Model file for the job. Use its own axes, mm. Face numbers are marked on the shaded views. A direction names the side the tool comes from. Give positions to 0.01 mm unless a question says otherwise; leave off trailing zeros. Order: outer loops, then holes, each group sorted by start corner. A loop starts at its lowest first (then second) coordinate and runs counter-clockwise, first axis right, second up. Notation, with made-up numbers: (87.25, -15.75) - (112.25, -15.75) arc R29 ccw to (112.25, 21.25) - close; hole circle Ø5 at (42, 80.25). An arc over 180 degrees is marked (long way). Return JSON: item names as keys, results as strings. Group by question number.
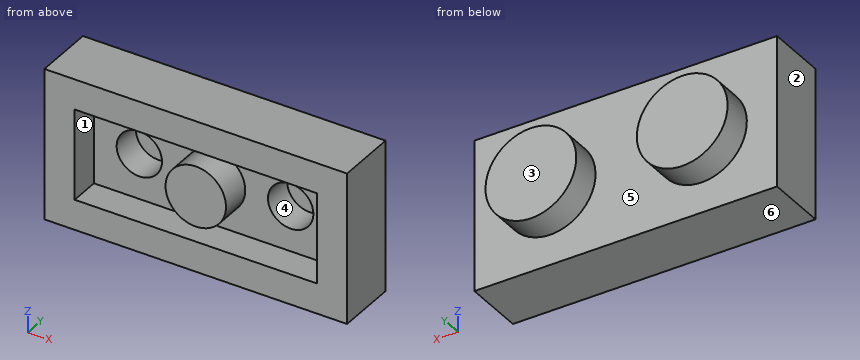
from build123d import *

# Parameters (mm, degrees)
SKETCH1_R           = 1.5
SKETCH1_R_2         = 0.75
BOSS_EXTRUDE1_DEPTH = 2
SKETCH1_3_W         = 10
SKETCH1_3_H         = 5
BOSS_EXTRUDE2_DEPTH = 1
SKETCH1_4_R         = 0.75
CUT_EXTRUDE1_DEPTH  = 1
SKETCH1_5_W         = 10
SKETCH1_5_H         = 5
SKETCH1_5_W_2       = 8
SKETCH1_5_H_2       = 3
SKETCH1_5_R         = 1
BOSS_EXTRUDE3_DEPTH = 1


with BuildPart() as part:
    # Sketch1 → Boss-Extrude1 (new body)
    with BuildSketch(Plane(origin=(0, 0, 0), x_dir=(1, 0, 0), z_dir=(0, 1, 0))):
        with Locations(Location((-2.5, 0, 0), (0, 0, 270))):
            Circle(SKETCH1_R)
        with Locations((-2.5, 0)):
            Circle(SKETCH1_R_2, mode=Mode.SUBTRACT)
        with Locations((-2.5, 0)):
            Circle(SKETCH1_R_2)
        with Locations(Location((2.5, 0, 0), (0, 0, 270))):
            Circle(SKETCH1_R)
        with Locations((2.5, 0)):
            Circle(SKETCH1_R_2, mode=Mode.SUBTRACT)
        with Locations((2.5, 0)):
            Circle(SKETCH1_R_2)
    extrude(amount=BOSS_EXTRUDE1_DEPTH)

    # Sketch1_3 → Boss-Extrude2 (add)
    with BuildSketch(Plane(origin=(0, 0, 0), x_dir=(1, 0, 0), z_dir=(0, 1, 0))):
        Rectangle(SKETCH1_3_W, SKETCH1_3_H)
    extrude(amount=BOSS_EXTRUDE2_DEPTH)

    # Sketch1_4 → Cut-Extrude1 (cut)
    with BuildSketch(Plane(origin=(0, 0, 0), x_dir=(1, 0, 0), z_dir=(0, 1, 0))):
        with Locations(Location((-2.5, 0, 0), (0, 0, 270))):
            Circle(SKETCH1_4_R)
        with Locations(Location((2.5, 0, 0), (0, 0, 270))):
            Circle(SKETCH1_4_R)
    extrude(amount=CUT_EXTRUDE1_DEPTH, mode=Mode.SUBTRACT)

    # Sketch1_5 → Boss-Extrude3 (add)
    with BuildSketch(Plane(origin=(0, 0, 0), x_dir=(1, 0, 0), z_dir=(0, 1, 0))):
        Rectangle(SKETCH1_5_W, SKETCH1_5_H)
        Rectangle(SKETCH1_5_W_2, SKETCH1_5_H_2, mode=Mode.SUBTRACT)
        with Locations(Location((0, 0, 0), (0, 0, 270))):
            Circle(SKETCH1_5_R)
    extrude(amount=-BOSS_EXTRUDE3_DEPTH)


solid = part.part
(1) Drill centre lines: L1, parallel to X at y = 0.7, z = 0; L2, parallel to Z at x = -1.75, y = -0.5; L3, parallel to X at y = 0.05, z = 0.4. Where is each one in solid material? Low to high.
(2) Slice it at A-A (y = -0.65). Give the cut face in (x, z), and give its area (3 significant figures).
(3) Drop flat-ended pins along their axis: pin 1 Ø0.9 at (x, z) = (-2.5, 0) entering from -Y; pin 2 Ø1 at (x, z) = (0, 2) entering from +Y; pin 3 Ø2 at (x, z) = (2.5, 0) entering from -Y. Give the stop position or say it passes through.
(4) Slice it at D-D (y = 0.45). Give the cut face in (x, z), and give its area (3 significant figures).
(5) Pull direction X, two halves, no side cores. Call the marked faces 1, 2 and 3: released by +X, released by -X, zero draft, split by the parting line, or undercut.
(6) Slice it at B-B (x = 0). Give the cut face in (y, z), and give its area (3 significant figures).
(7) 3-axis set-ups, long thin cutter, end or side, ignore diameter. For the marked faces 4, 5 and 6: which of +Z, -Z, +X, -X, +Y, -Y reach the whole face in a straight line?
(8) Slice it at C-C (z = 0). Give the cut face in (x, y), and give its area (3 significant figures).
Result set:
{
 "1": {"L1": "x = -5 to -3.25, -1.75 to 1.75, 3.25 to 5", "L2": "z = -2.5 to -1.5, 1.5 to 2.5", "L3": "x = -5 to -3.13, -1.87 to 1.87, 3.13 to 5"},
 "2": {"outline": "(-5, -2.5) - (5, -2.5) - (5, 2.5) - (-5, 2.5) - close; circle Ø2 at (0, 0); hole (-4, -1.5) - (4, -1.5) - (4, 1.5) - (-4, 1.5) - close", "area": "29.1 mm²"},
 "3": {"pin 1": "stops at y = 1", "pin 2": "stops at y = 1", "pin 3": "stops at y = 0"},
 "4": {"outline": "(-5, -2.5) - (5, -2.5) - (5, 2.5) - (-5, 2.5) - close; hole circle Ø1.5 at (-2.5, 0); hole circle Ø1.5 at (2.5, 0)", "area": "46.5 mm²"},
 "5": {"face 1": "undercut", "face 2": "released by -X", "face 3": "zero draft"},
 "6": {"outline": "(-1, -2.5) - (1, -2.5) - (1, 2.5) - (-1, 2.5) - (-1, 1.5) - (0, 1.5) - (0, 1) - (-1, 1) - (-1, -1) - (0, -1) - (0, -1.5) - (-1, -1.5) - close", "area": "9.00 mm²"},
 "7": {"face 4": "-Y", "face 5": "+Y", "face 6": "-Z, +X, -X, +Y, -Y"},
 "8": {"outline": "(-5, -1) - (-4, -1) - (-4, 0) - (-3.25, 0) - (-3.25, 1) - (-1.75, 1) - (-1.75, 0) - (-1, 0) - (-1, -1) - (1, -1) - (1, 0) - (1.75, 0) - (1.75, 1) - (3.25, 1) - (3.25, 0) - (4, 0) - (4, -1) - (5, -1) - (5, 1) - (4, 1) - (4, 2) - (1, 2) - (1, 1) - (-1, 1) - (-1, 2) - (-4, 2) - (-4, 1) - (-5, 1) - close", "area": "17.0 mm²"}
}
